Source: three-view drawing plus pictorial views. Frame: mm from the lowest corner of the part. Round coordinates to 2 decimals unless told otherwise and drop trailing zeros. Loops run counter-clockwise (first coordinate to the right, second up) from the corner with the lowest first, then second, coordinate; pieces in that order, holes last. Notation, with made-up numbers: M 44,-1 L 58,-1 A17 ccw 58,20 Z; hole C -27.5,23 d7. An arc over 180 degrees is marked long. Answer as a JSON object with one key per item and string values.
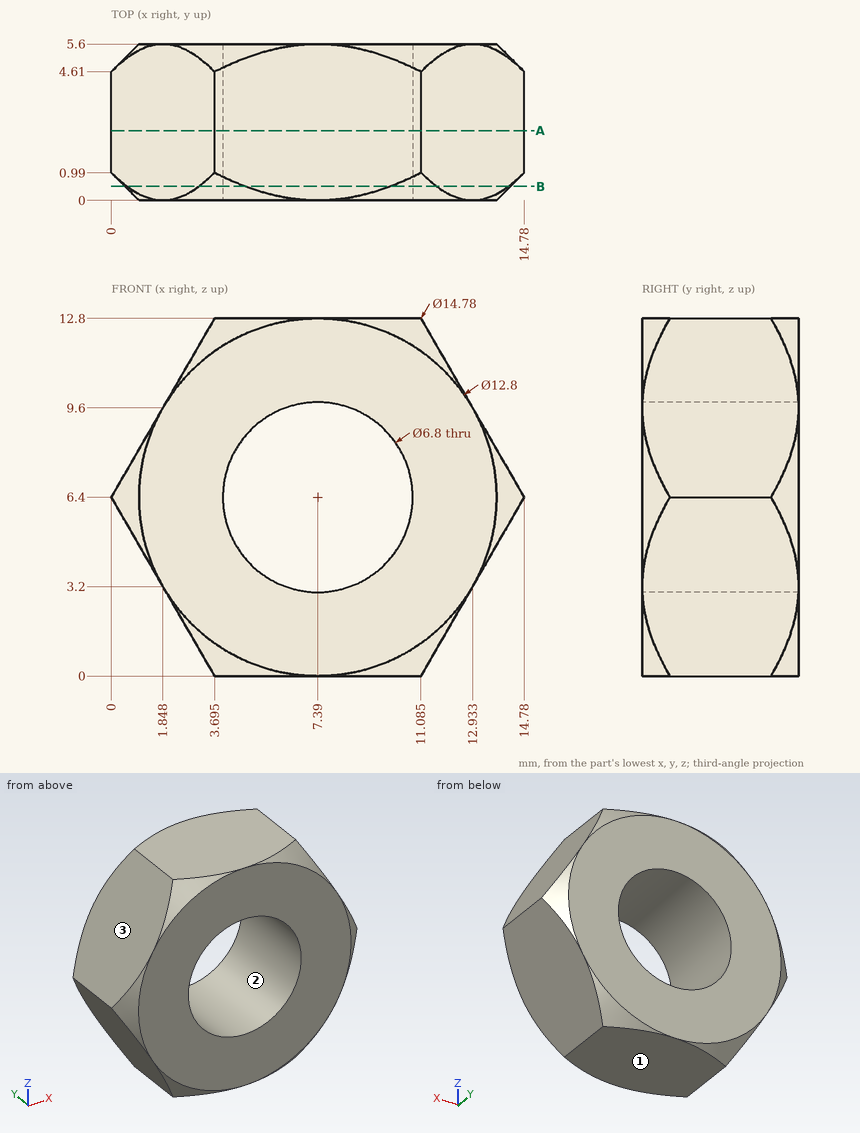
1) First-contact query: pin 1 (1.5 mm diameter, centred on y = 3.5, z = 11, fed in from +X); pin 2 (2 mm diameter, centred on y = 3, z = 8.5, fed in from +X) (1 decimal); pin 3 (3 mm diameter, centred on y = 1.5, z = 4.5, fed in from -X). Flat tips, straight axial feed; report the tip coordinate or a pass-through.
Geometry results:
{"pin 1": "x = 12.56", "pin 2": "x = 14.1", "pin 3": "x = 0.23"}
2) Cut plane B-B on y = 0.5. Return the cut outline in (x, z).
Geometry results:
{"outline": "M 0.56,5.43 L 3.14,0.97 A6.9 ccw 4.81,0 L 9.97,0 A6.9 ccw 11.64,0.97 L 14.22,5.43 A6.9 ccw 14.22,7.37 L 11.64,11.83 A6.9 ccw 9.97,12.8 L 4.81,12.8 A6.9 ccw 3.14,11.83 L 0.56,7.37 A6.9 ccw Z; hole C 7.39,6.4 d6.8"}
3) Pull-direction query (X, two-part tool) for the marked faces 1, 2 and 3; classes: +X half, -X half, draft (parallel to the pull), parting line (faces both ways), or undercut.
Geometry results:
{"face 1": "draft", "face 2": "undercut", "face 3": "-X half"}
4) Cut plane A-A on y = 2.5. Return the cut outline in (x, z) (1 decimal), and give its area (3 significant figures).
Geometry results:
{"outline": "M 0,6.4 L 3.7,0 L 11.1,0 L 14.8,6.4 L 11.1,12.8 L 3.7,12.8 Z; hole C 7.4,6.4 d6.8", "area": "106 mm2"}
5) Line query: probe 1 along Z at (x, y) = (5.75, 3.4); probe 2 along X at (y, z) = (4.3, 7.75); probe 3 along X at (y, z) = (1.5, 5.5). Output: solid intervals per line, ascending.
Geometry results:
{"probe 1": "0 to 3.42, 9.38 to 12.8", "probe 2": "0.78 to 4.27, 10.51 to 14", "probe 3": "0.52 to 4.11, 10.67 to 14.26"}
